The listing builds one solid part. Answer for the finished solid, in the listing's coordinates (mm). Face numbers are marked on the shaded views. A direction names the side the tool comes from. Round coordinates to 2 decimals unless told otherwise and drop trailing zeros.
from build123d import *

# Parameters (mm, degrees)
F1_DEPTH     = 6.35
F2_R         = 11.049
F3_DEPTH     = 25.4
F5_DEPTH     = 25.4
F7_DEPTH     = 25.4
F8_T2_ANGLE  = 244.4198027275
F8_T4_ANGLE  = 244.4198027276
F8_T6_ANGLE  = 244.4198027276
F8_T8_ANGLE  = 244.4198027276
F8_T10_ANGLE = 244.4198027275
F8_T12_ANGLE = 244.4198027276
F9_R         = 11.2522
F10_DEPTH    = 25.4
F12_DEPTH    = 25.4


# Not quite as in the source:
# - a fillet or chamfer that OpenCascade refuses, or shapes differently, is made with other operations: its cross-section is extruded or revolved along the edge and cut away or added


with BuildPart() as f1:
    # F0 (on Top) → F1 (new body)
    with BuildSketch(Plane.XY):
        with BuildLine():
            ThreePointArc((25.4522914495, -0.5462737247), (25.4566875826, -0.2731525857), (25.4581530165, 0))
            ThreePointArc((25.4581530165, 0), (24.3796049896, 7.3316038874), (21.2353474165, 14.0419932742))
            ThreePointArc((21.2353474165, 14.0419932742), (21.1161182893, 14.2149891818), (21.000703446, 14.3905527964))
            ThreePointArc((21.000703446, 14.3905527964), (5.9018125459, 24.7646151532), (-12.2530588017, 22.3154678422))
            ThreePointArc((-12.2530588017, 22.3154678422), (-18.3508874647, 17.6454663942), (-22.7783966035, 11.3693536837))
            ThreePointArc((-22.7783966035, 11.3693536837), (-22.8686008906, 11.1796002769), (-22.9629360192, 10.9918662834))
            ThreePointArc((-22.9629360192, 10.9918662834), (-24.3976921105, -7.2711879835), (-13.1992326478, -21.7691941174))
            ThreePointArc((-13.1992326478, -21.7691941174), (-6.1059784266, -24.7150679236), (1.543049187, -25.411346958))
            ThreePointArc((1.543049187, -25.411346958), (1.7524826013, -25.3945894587), (1.9622325732, -25.3824190798))
            ThreePointArc((1.9622325732, -25.3824190798), (18.4958795647, -17.4934271697), (25.4522914495, -0.5462737247))
        make_face()
        with BuildLine():
            ThreePointArc((-40.840152687, 13.2027706404), (-32.3672544542, -8.5097837592), (-13.1992326478, -21.7691941174))
            ThreePointArc((-13.1992326478, -21.7691941174), (-24.3976921105, -7.2711879835), (-22.9629360192, 10.9918662834))
            ThreePointArc((-22.9629360192, 10.9918662834), (-32.671913716, 5.8681661373), (-40.840152687, 13.2027706404))
        make_face()
        with BuildLine():
            ThreePointArc((-12.2530588017, 22.3154678422), (5.9018125459, 24.7646151532), (21.000703446, 14.3905527964))
            ThreePointArc((21.000703446, 14.3905527964), (21.4179378065, 25.3606241997), (31.8540111184, 28.7672244012))
            ThreePointArc((31.8540111184, 28.7672244012), (8.8139383109, 32.2857564877), (-12.2530588017, 22.3154678422))
        make_face()
        with BuildLine():
            ThreePointArc((8.9861415686, -41.9699950416), (23.5533161433, -23.7759727285), (25.4522914495, -0.5462737247))
            ThreePointArc((25.4522914495, -0.5462737247), (18.4958795647, -17.4934271697), (1.9622325732, -25.3824190798))
            ThreePointArc((1.9622325732, -25.3824190798), (11.2539759095, -31.2287903369), (8.9861415686, -41.9699950416))
        make_face()
    extrude(amount=F1_DEPTH)

    # F2 (on face) → F3 (cut)
    with BuildSketch(Plane(origin=(0, 0, 0), x_dir=(1, 0, 0), z_dir=(0, 0, -1))):
        Circle(F2_R)
    extrude(amount=-F3_DEPTH, mode=Mode.SUBTRACT)

    # F4 (on face) → F5 (cut)
    with BuildSketch(Plane(origin=(0, 0, 0), x_dir=(1, 0, 0), z_dir=(0, 0, -1))):
        with BuildLine():
            ThreePointArc((-15.9673679457, 5.2488333315), (-5.0596183633, 16.0283296844), (10.0600734805, 13.4648435572))
            Line((10.0600734805, 13.4648435572), (13.19237559, 17.0424425012))
            ThreePointArc((13.19237559, 17.0424425012), (-6.5891713979, 20.5199035183), (-20.6480469686, 6.1759028892))
            Line((-20.6480469686, 6.1759028892), (-15.9673679457, 5.2488333315))
        make_face()
        with BuildLine():
            ThreePointArc((12.5293069781, 11.2037296068), (15.7018951262, 5.9964639497), (16.8079472409, 0))
            ThreePointArc((16.8079472409, 0), (14.03492488, -9.2481335449), (6.6308598383, -15.4447009767))
            Line((6.6308598383, -15.4447009767), (8.1630003536, -19.9461536478))
            ThreePointArc((8.1630003536, -19.9461536478), (17.8942957524, -12.0115694078), (21.551882055, 0))
            ThreePointArc((21.551882055, 0), (20.0281771041, 7.9596320267), (15.6725122776, 14.7937817687))
            Line((15.6725122776, 14.7937817687), (12.5293069781, 11.2037296068))
        make_face()
        with BuildLine():
            Line((4.975534691, -20.9696846579), (3.4380609675, -16.4525629383))
            ThreePointArc((3.4380609675, -16.4525629383), (-11.3511315053, -12.3959228782), (-16.6909333188, 1.9798574195))
            Line((-16.6909333188, 1.9798574195), (-21.3553759436, 2.9037111466))
            ThreePointArc((-21.3553759436, 2.9037111466), (-14.4761720311, -15.9663415797), (4.975534691, -20.9696846579))
        make_face()
    extrude(amount=-F5_DEPTH, mode=Mode.SUBTRACT)

    # F6 (on face) → F7 (cut)
    with BuildSketch(Plane(origin=(0, 0, 0), x_dir=(1, 0, 0), z_dir=(0, 0, -1))):
        with BuildLine():
            Line((-31.5523461387, -2.6979510549), (-31.5523461387, 5.8615701514))
            ThreePointArc((-31.5523461387, 5.8615701514), (-34.8955742826, 1.5818095483), (-31.5523461387, -2.6979510549))
        make_face()
        with BuildLine():
            ThreePointArc((-29.303277888, -2.6679827758), (-26.9727125071, -1.0870330259), (-26.0737039307, 1.5818095483))
            ThreePointArc((-26.0737039307, 1.5818095483), (-26.9727125071, 4.2506521224), (-29.303277888, 5.8316018723))
            Line((-29.303277888, 5.8316018723), (-29.303277888, -2.6679827758))
        make_face()
        with BuildLine():
            ThreePointArc((20.8524417265, 24.3943482294), (20.9802584593, 24.9959924433), (21.023141982, 25.6095671174))
            ThreePointArc((21.023141982, 25.6095671174), (18.2648613778, 29.6991981513), (13.4396789177, 28.6741088325))
            Line((13.4396789177, 28.6741088325), (20.8524417265, 24.3943482294))
        make_face()
        with BuildLine():
            Line((19.7019543101, 22.461582129), (12.3410980833, 26.711374453))
            ThreePointArc((12.3410980833, 26.711374453), (14.4067392181, 21.7895852006), (19.7019543101, 22.461582129))
        make_face()
        with BuildLine():
            Line((9.6013235778, -28.2931840013), (16.9621798046, -24.0433916772))
            ThreePointArc((16.9621798046, -24.0433916772), (11.6669647126, -23.3713947489), (9.6013235778, -28.2931840013))
        make_face()
        with BuildLine():
            ThreePointArc((10.6999044122, -30.2559183808), (15.5250868723, -31.2810076995), (18.2833674765, -27.1913766657))
            ThreePointArc((18.2833674765, -27.1913766657), (18.2404839539, -26.5778019915), (18.112667221, -25.9761577777))
            Line((18.112667221, -25.9761577777), (10.6999044122, -30.2559183808))
        make_face()
    extrude(amount=-F7_DEPTH, mode=Mode.SUBTRACT)

    # F8: fillet of radius 2.54 on 6 edges, made by hand

    # F8_s1 → F8_t2 (revolve, cut)
    with BuildSketch(Plane(origin=(-16.1639945801, -15.1453497234, 0), x_dir=(0, 0, 1), z_dir=(-0.7297262835, -0.6837393883, 0))):
        with BuildLine():
            ThreePointArc((6.35, -15.029889874), (5.6060512242, -16.8259410982), (3.81, -17.569889874))
            Line((3.81, -17.569889874), (6.35, -17.569889874))
            Line((6.35, -17.569889874), (6.35, -15.029889874))
        make_face()
    revolve(axis=Axis((2.4134385694, -34.9722625532, 6.35), (0, 0, -1)), revolution_arc=F8_T2_ANGLE, mode=Mode.SUBTRACT)

    # F8_s3 → F8_t4 (revolve, cut)
    with BuildSketch(Plane(origin=(-5.0342603196, 21.5711047947, 0), x_dir=(0, 0, 1), z_dir=(-0.2272725381, 0.9738311935, 0))):
        with BuildLine():
            ThreePointArc((6.35, -15.029889874), (5.6060512242, -16.8259410982), (3.81, -17.569889874))
            Line((3.81, -17.569889874), (6.35, -17.569889874))
            Line((6.35, -17.569889874), (6.35, -15.029889874))
        make_face()
    revolve(axis=Axis((-31.4935870836, 15.396032165, 6.35), (0, 0, -1)), revolution_arc=F8_T4_ANGLE, mode=Mode.SUBTRACT)

    # F8_s5 → F8_t6 (revolve, cut)
    with BuildSketch(Plane(origin=(21.1982548997, -6.4257550714, 0), x_dir=(0, 0, 1), z_dir=(0.9569988216, -0.2900918052, 0))):
        with BuildLine():
            ThreePointArc((3.81, -17.569889874), (5.6060512242, -16.8259410982), (6.35, -15.029889874))
            Line((6.35, -15.029889874), (6.35, -17.569889874))
            Line((6.35, -17.569889874), (3.81, -17.569889874))
        make_face()
    revolve(axis=Axis((29.0801485142, 19.5762303882, 6.35), (0, 0, -1)), revolution_arc=F8_T6_ANGLE, mode=Mode.SUBTRACT)

    # F8_s7 → F8_t8 (revolve, cut)
    with BuildSketch(Plane(origin=(-5.0342603196, 21.5711047947, 0), x_dir=(0, 0, 1), z_dir=(-0.2272725381, 0.9738311935, 0))):
        with BuildLine():
            ThreePointArc((0, -15.029889874), (0.7439487758, -16.8259410982), (2.54, -17.569889874))
            Line((2.54, -17.569889874), (0, -17.569889874))
            Line((0, -17.569889874), (0, -15.029889874))
        make_face()
    revolve(axis=Axis((-31.4935870836, 15.396032165, 0), (0, 0, -1)), revolution_arc=F8_T8_ANGLE, mode=Mode.SUBTRACT)

    # F8_s9 → F8_t10 (revolve, cut)
    with BuildSketch(Plane(origin=(-16.1639945801, -15.1453497234, 0), x_dir=(0, 0, 1), z_dir=(-0.7297262835, -0.6837393883, 0))):
        with BuildLine():
            ThreePointArc((0, -15.029889874), (0.7439487758, -16.8259410982), (2.54, -17.569889874))
            Line((2.54, -17.569889874), (0, -17.569889874))
            Line((0, -17.569889874), (0, -15.029889874))
        make_face()
    revolve(axis=Axis((2.4134385694, -34.9722625532, 0), (0, 0, -1)), revolution_arc=F8_T10_ANGLE, mode=Mode.SUBTRACT)

    # F8_s11 → F8_t12 (revolve, cut)
    with BuildSketch(Plane(origin=(21.1982548997, -6.4257550714, 0), x_dir=(0, 0, 1), z_dir=(0.9569988216, -0.2900918052, 0))):
        with BuildLine():
            ThreePointArc((2.54, -17.569889874), (0.7439487758, -16.8259410982), (0, -15.029889874))
            Line((0, -15.029889874), (0, -17.569889874))
            Line((0, -17.569889874), (2.54, -17.569889874))
        make_face()
    revolve(axis=Axis((29.0801485142, 19.5762303882, 0), (0, 0, -1)), revolution_arc=F8_T12_ANGLE, mode=Mode.SUBTRACT)

    # F9 (on Top) → F10 (cut)
    with BuildSketch(Plane.XY):
        Circle(F9_R)
    extrude(amount=-F10_DEPTH, mode=Mode.SUBTRACT)

    # F11 (on face) → F12 (cut)
    with BuildSketch(Plane.XY.offset(6.35)):
        Polygon((6.5367808275, 29.8250825475), (6.0469240758, 30.6364076297), (-6.8415322731, 25.3754631249), (-6.3712364353, 24.5042187493), align=None)
        Polygon((7.6234762433, 28.0252436261), (7.1763426779, 28.7658084453), (-5.8592754632, 23.5557878219), (-5.3787292375, 22.6655541377), align=None)
        Polygon((22.5608887424, -20.5735595293), (23.5084452502, -20.5549936793), (25.3965618355, -6.7627908131), (24.4068941544, -6.7344567681), align=None)
        Polygon((20.4588348058, -20.6147459049), (21.3237495351, -20.597799288), (23.3295483915, -6.7036125121), (22.3183102928, -6.6746609091), align=None)
        Polygon((-29.0976695699, -9.2515230182), (-29.5553693259, -10.0814139505), (-18.5550295624, -18.6126723118), (-18.0356577191, -17.7697619811), align=None)
        Polygon((-28.0823110491, -7.4104977212), (-28.500092213, -8.1680091574), (-17.4702729283, -16.8521753098), (-16.9395810553, -15.9908932286), align=None)
    extrude(amount=-F12_DEPTH, mode=Mode.SUBTRACT)


solid = f1.part
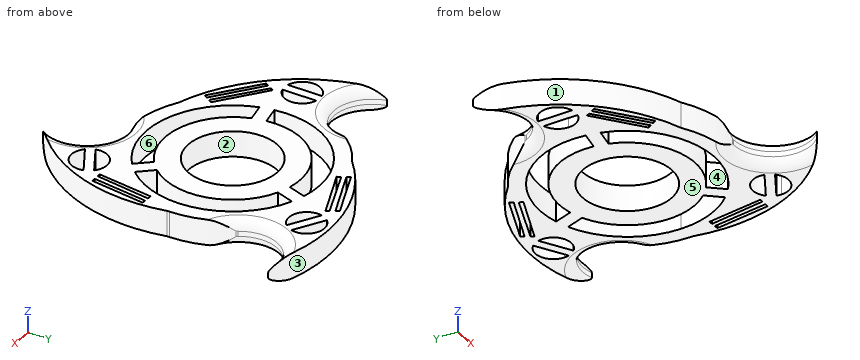
1. Given pin 1 (3 mm diameter, centred on y = -3, z = 2.5, fed in from +X); pin 2 (1 mm diameter, centred on x = 24, z = 2.5, fed in from +Y); pin 3 (1.5 mm diameter, centred on x = -19, z = 4.5, fed in from -Y), each flat-ended and moving along its own axis, determine where each tip first touches the part or whether it passes through.
Geometry says:
pin 1: stops at x = 26.11
pin 2: stops at y = 31.69
pin 3: stops at y = -19.77
2. A tool of negligible diameter and unlimited length cuts with its end or side. For the marked faces 5 and 6, from which of +Z, -Z, +X, -X, +Y, -Y can it reach the whole face along a straight path? Write none if from no direction.
Geometry says:
face 5: -Z, +X, -X, +Y, -Y
face 6: +Z, -Z
3. Straight lines are drawn through the part: line 1 along Y through (x, z) = (2, 0.5); line 2 along X through (y, z) = (7, 1.75); line 3 along X through (y, z) = (13, 6). For each, find the intervals that lie inside material, in ascending order.
Geometry says:
line 1: y = -24.35 to -21.46, -16.69 to -10.87, 10.87 to 16.69, 21.46 to 25.71, 26.7 to 27.95, 28.98 to 30.67
line 2: x = -39.88 to -36.4, -26.58 to -20.38, -15.28 to -8.55, 8.55 to 15.28, 20.38 to 24.48
line 3: x = -20.91 to -17.19, -10.65 to 10.65, 17.19 to 20.45
4. For a pull along X with two mould halves and no side action, classify the marked faces 1, 2, 3 and 4 as released by +X, released by -X, zero draft, split by the parting line, or undercut.
Geometry says:
face 1: released by -X
face 2: undercut
face 3: split by the parting line
face 4: undercut
5. Section A-A on x = 0 is taken. Give the number of separate pieces and of enclosed holes in the cut face, plus the area to 3 significant figures.
Geometry says:
separate pieces: 6
enclosed holes: 0
area: 136 mm2
